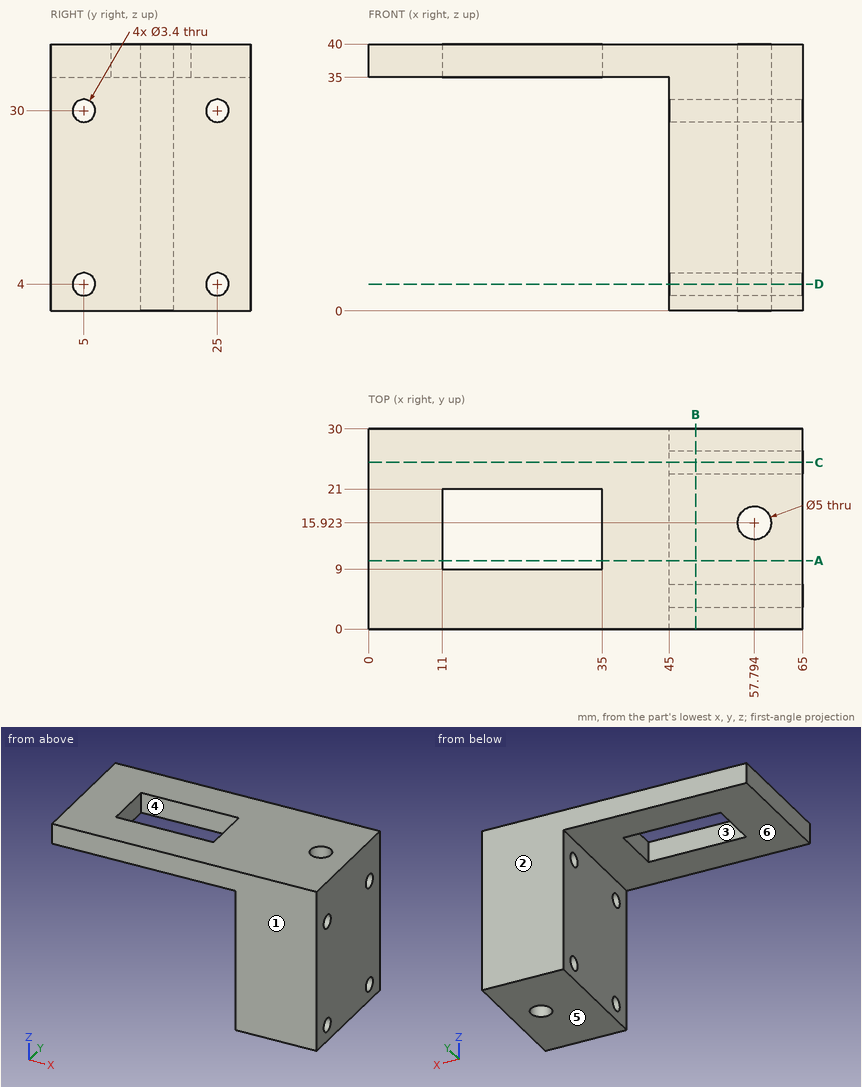
Can you work these out from the drawing? Everything is in mm from the part's minimum corner. A direction names the side the tool comes from. Give positions to 0.01 mm unless a question says otherwise; leave off trailing zeros. Order: outer loops, then holes, each group sorted by start corner. A loop starts at its lowest first (then second) coordinate and runs counter-clockwise, first axis right, second up.
1. For the marked faces 5 and 6, which set-ups out of +Z, -Z, +X, -X, +Y, -Y let a thin tool reach every point of the face, with its end or its side?
2. Suppose I cut it at D-D (z = 4). List the corners of the cut face in (x, y) for me.
3. Suppose I cut it at C-C (y = 25). List the corners of the cut face in (x, z) for me, plus the area to 3 significant figures.
4. Will these pins go through, and if not, where does the flat tip stop? P1, Ø15, axis at x = 20.5, y = 19, coming from the -Z side; P2, Ø1.5, axis at x = 18.5, z = 38, coming from the -Y side; P3, Ø4.5, axis at y = 5, z = 4, coming from the -X side; P4, Ø2, axis at y = 5, z = 30, coming from the +X side.
5. I need wall thicknesses on L1, parallel to Y at x = 58, z = 4; L2, parallel to Y at x = 55, z = 4; L3, parallel to Y at x = 57, z = 4. Which ranges of each line are inside material? Lowest first, please.
6. Suppose I cut it at A-A (y = 10.25). List the corners of the cut face in (x, z) for me.
7. We'd pull the mould along Y, two halves only. Please class the marked faces 1, 2, 3 and 4: pulls with the +Y half, pulls with the -Y half, needs draft (parallel to the pull), parting line crosses it, or undercut.
8. Suppose I cut it at B-B (x = 49). List the corners of the cut face in (y, z) for me.
Solved:
1. face 5: -Z, +X, -X, +Y, -Y
1. face 6: -Z, -X, +Y, -Y
2. outline: (45, 0) - (65, 0) - (65, 3.3) - (45, 3.3) - close; (45, 6.7) - (65, 6.7) - (65, 23.3) - (45, 23.3) - close; (45, 26.7) - (65, 26.7) - (65, 30) - (45, 30) - close; hole circle Ø5 at (57.79, 15.92)
3. outline: (0, 35) - (45, 35) - (45, 31.7) - (65, 31.7) - (65, 40) - (0, 40) - close; (45, 0) - (65, 0) - (65, 2.3) - (45, 2.3) - close; (45, 5.7) - (65, 5.7) - (65, 28.3) - (45, 28.3) - close
3. area: 889 mm2
4. P1: stops at z = 35
4. P2: stops at y = 0
4. P3: stops at x = 45
4. P4: passes through
5. L1: y = 0 to 3.3, 6.7 to 13.43, 18.41 to 23.3, 26.7 to 30
5. L2: y = 0 to 3.3, 6.7 to 23.3, 26.7 to 30
5. L3: y = 0 to 3.3, 6.7 to 13.55, 18.29 to 23.3, 26.7 to 30
6. outline: (0, 35) - (11, 35) - (11, 40) - (0, 40) - close; (35, 35) - (45, 35) - (45, 0) - (65, 0) - (65, 40) - (35, 40) - close
7. face 1: pulls with the -Y half
7. face 2: pulls with the +Y half
7. face 3: undercut
7. face 4: undercut
8. outline: (0, 0) - (30, 0) - (30, 40) - (0, 40) - close; hole circle Ø3.4 at (5, 4); hole circle Ø3.4 at (5, 30); hole circle Ø3.4 at (25, 4); hole circle Ø3.4 at (25, 30)
